from build123d import *

# Parameters (mm, degrees)
SKETCH3_W           = 393.7
SKETCH3_H           = 76.2
BOSS_EXTRUDE1_DEPTH = 6.35
SKETCH4_R           = 3.175
CUT_EXTRUDE1_DEPTH  = 6.35
SKETCH6_R           = 3.175
CUT_EXTRUDE3_DEPTH  = 6.35


with BuildPart() as part:
    # Sketch3 → Boss-Extrude1 (new body)
    with BuildSketch(Plane(origin=(0, 0, 0), x_dir=(0, 0, -1), z_dir=(1, 0, 0))):
        Rectangle(SKETCH3_W, SKETCH3_H)
    extrude(amount=BOSS_EXTRUDE1_DEPTH)

    # Sketch4 → Cut-Extrude1 (cut)
    with BuildSketch(Plane.ZY):
        with Locations((181.85, 0)):
            Circle(SKETCH4_R)
    extrude(amount=-CUT_EXTRUDE1_DEPTH, mode=Mode.SUBTRACT)

    # Sketch6 → Cut-Extrude3 (cut)
    with BuildSketch(Plane.ZY):
        with Locations((-184.15, 0)):
            Circle(SKETCH6_R)
    extrude(amount=-CUT_EXTRUDE3_DEPTH, mode=Mode.SUBTRACT)


solid = part.part
Verification items for the finished model (mm, model axes). Coordinates: 2 decimals unless noted, no trailing zeros. Use CSV: the item, a comma, the result in double quotes.
Q1. Go/stop test with flat-tipped pins: P1, Ø5, axis at y = 0, z = -184.15, coming from the -X side; P2, Ø7.5, axis at y = 0, z = 181.85, coming from the -X side. Record where each tip stops, or that it passes through.
Computed values:
P1,"through"
P2,"x = 0"
Q2. Thickness scan on line 1 along Y through (x, z) = (4, 181.85) (3 decimals). Record the ranges inside material, lowest first. Write a range as [from, to].
Computed values:
line 1,"[-38.1, -3.175], [3.175, 38.1]"
Q3. Mould release check, pull along Y, two halves, no side actions. Record for faces 1 (the flat face through (3, 38.1, 3)), 2 (the cylindrical face through (3.13, -1.22, -181.22)), 3 (the flat face through (3, -1, -196.85)): pulls with the +Y half, pulls with the -Y half, needs draft (parallel to the pull), parting line crosses it, or undercut.
Computed values:
face 1,"pulls with the +Y half"
face 2,"undercut"
face 3,"needs draft"
